Drawing for the job (mm, zero at the part's lowest x, y, z). A direction names the side the tool comes from. Round coordinates to 2 decimals unless told otherwise and drop trailing zeros. Loops run counter-clockwise (first coordinate to the right, second up) from the corner with the lowest first, then second, coordinate; pieces in that order, holes last. Notation, with made-up numbers: M 14.25,32 L 51.25,32 A36 cw 51.25,68 Z; hole C 75.25,56 d3. An arc over 180 degrees is marked long. Answer in a Markdown table with one row per item.
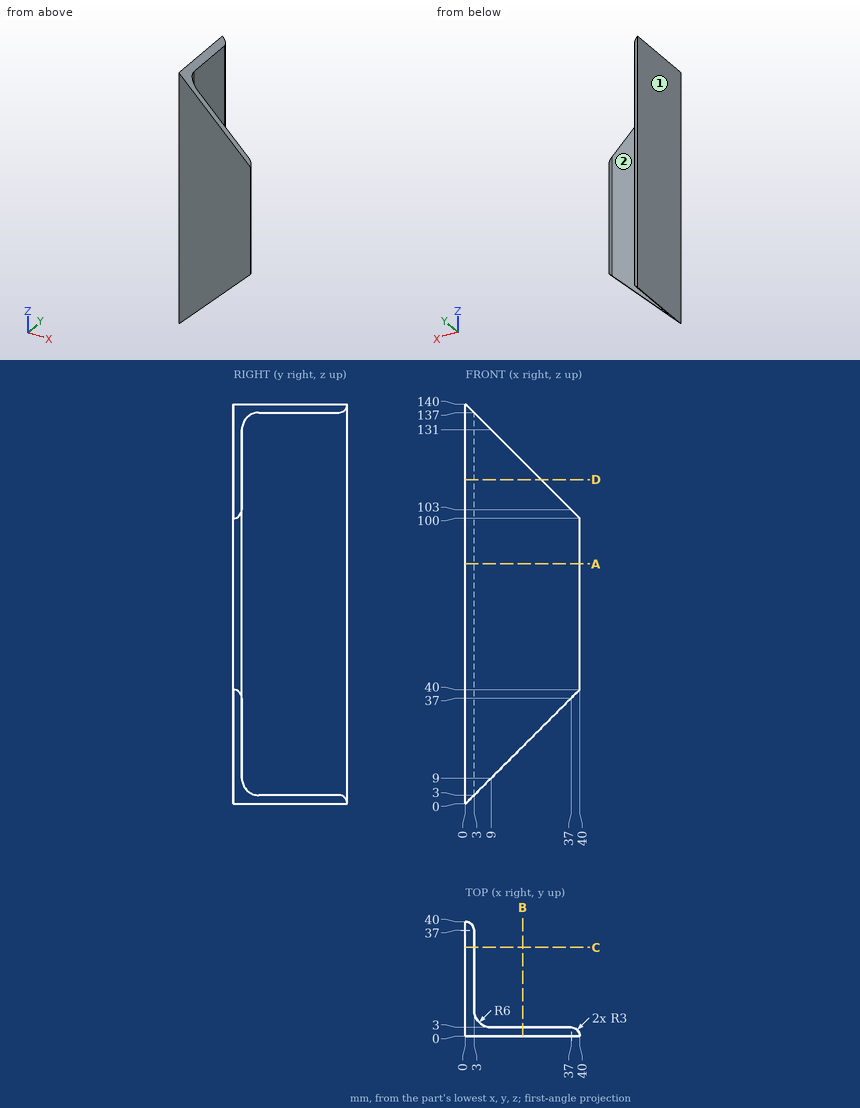
1. Wall check: probe 1 along X at (y, z) = (15, 18); probe 2 along Y at (x, z) = (4, 98). Give the ranges that are in metal, low to high.
Verdict:
| item | result |
|---|---|
| probe 1 | x = 0 to 3 |
| probe 2 | y = 0 to 5.68 |
2. Saw through at A-A (z = 84). Write the cut outline in (x, y), and give its area (3 significant figures).
Verdict:
| item | result |
|---|---|
| outline | M 0,0 L 40,0 A3 ccw 37,3 L 9,3 A6 cw 3,9 L 3,37 A3 ccw 0,40 Z |
| area | 235 mm² |
3. Tool access for the marked faces 1 and 2: list every direction of +Z, -Z, +X, -X, +Y, -Y with a clear straight run to the whole face (end or side of a thin tool).
Verdict:
| item | result |
|---|---|
| face 1 | +Z, -Z, -X, +Y, -Y |
| face 2 | +Z, -Z, +X, +Y |
4. Pin check, flat tips, straight feed: pin 1 (10 mm diameter, centred on x = 8.5, z = 82, fed in from +Y); pin 2 (10 mm diameter, centred on x = 13.5, z = 61.5, fed in from +Y); pin 3 (8.5 mm diameter, centred on y = 20, z = 84, fed in from +X). Stop position of each tip, or through.
Verdict:
| item | result |
|---|---|
| pin 1 | stops at y = 6.6 |
| pin 2 | stops at y = 3.02 |
| pin 3 | stops at x = 3 |
5. Saw through at D-D (z = 113.5). Write the cut outline in (x, y).
Verdict:
| item | result |
|---|---|
| outline | M 0,0 L 26.5,0 L 26.5,3 L 9,3 A6 cw 3,9 L 3,37 A3 ccw 0,40 Z |
6. Saw through at B-B (x = 20). Write the cut outline in (y, z), and give its area (3 significant figures).
Verdict:
| item | result |
|---|---|
| outline | M 0,20 L 3,20 L 3,120 L 0,120 Z |
| area | 300 mm² |
7. Saw through at C-C (y = 31). Write the cut outline in (x, z).
Verdict:
| item | result |
|---|---|
| outline | M 0,0 L 3,3 L 3,137 L 0,140 Z |
